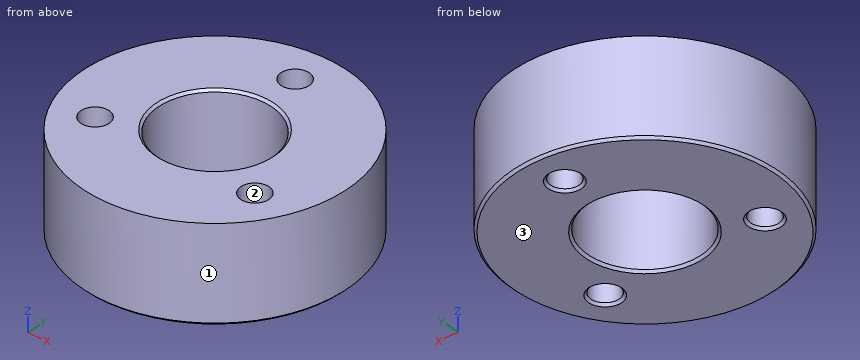
```python
from build123d import *

# Parameters (mm, degrees)
SKETCH2_R           = 14
SKETCH2_R_2         = 6
SKETCH2_R_3         = 1.5
BOSS_EXTRUDE1_DEPTH = 10
CHAMFER1_SIZE       = 0.25


with BuildPart() as part:
    # Sketch2 → Boss-Extrude1 (new body)
    with BuildSketch(Plane.XY):
        Circle(SKETCH2_R)
        Circle(SKETCH2_R_2, mode=Mode.SUBTRACT)
        with Locations((0, 10)):
            Circle(SKETCH2_R_3, mode=Mode.SUBTRACT)
        with Locations((8.660254038, -5)):
            Circle(SKETCH2_R_3, mode=Mode.SUBTRACT)
        with Locations((-8.660254038, -5)):
            Circle(SKETCH2_R_3, mode=Mode.SUBTRACT)
    extrude(amount=BOSS_EXTRUDE1_DEPTH)

    # Chamfer1
    chamfer1_edges = [part.edges().sort_by_distance(p)[0] for p in [
        (7.160254038, -5, 0),
        (-10.160254038, -5, 0),
        (-14, 0, 0),
        (-6, 0, 0),
        (-6, 0, 10),
        (-1.5, 10, 0),
    ]]
    chamfer(chamfer1_edges, length=CHAMFER1_SIZE)


solid = part.part
```
Check sheet for the modelled part. Datum: model origin and axes. Units: mm. Face numbers are marked on the shaded views. Give positions to 0.01 mm unless a question says otherwise; leave off trailing zeros. Order: outer loops, then holes, each group sorted by start corner. A loop starts at its lowest first (then second) coordinate and runs counter-clockwise, first axis right, second up. Notation, with made-up numbers: (-32, 76.5) -> (27, 76.5) arc R23 cw to (27, 90.5) -> close; hole circle Ø4 at (-12, -5). An arc over 180 degrees is marked (long way). Use CSV: the item, a comma, the result in double quotes. Start each with the question number.
1) Material ranges on line 1 (Y direction, x = 0, z = 4.5); line 2 (Y direction, x = -10, z = 1.75); line 3 (X direction, y = 1.5, z = 6), recorded low to high. Write a range as from..to.
2) Sectioned sample at A-A, the plane x = 0. Record the boundary of the cut face in (y, z).
3) Sectioned sample at B-B, the plane y = 0. Record the boundary of the cut face in (x, z), plus the area to 3 significant figures.
4) Sectioned sample at C-C, the plane z = 3.25. Record the boundary of the cut face in (x, y).
5) Sectioned sample at D-D, the plane y = -5. Give the number of separate pieces and of enclosed holes in the cut face, plus the area to 3 significant figures.
6) Mould release check, pull along X, two halves, no side actions. Record for the marked faces 1, 2 and 3: released by +X, released by -X, zero draft, split by the parting line, or undercut.
7) Go/stop test with flat-tipped pins: P1, Ø15.5, axis at x = 0, y = 0, coming from the +Z side; P2, Ø2.5, axis at x = 8.66, y = -5, coming from the +Z side; P3, Ø5, axis at y = -7, z = 3.5, coming from the +X side. Record where each tip stops, or that it passes through.
Recorded:
1,line 1,"-14..-6, 6..8.5, 11.5..14"
1,line 2,"-9.8..-5.67, -4.33..9.8"
1,line 3,"-13.92..-5.81, 5.81..13.92"
2,outline,"(-14, 0.25) -> (-13.75, 0) -> (-6.25, 0) -> (-6, 0.25) -> (-6, 9.75) -> (-6.25, 10) -> (-14, 10) -> close; (6, 0.25) -> (6.25, 0) -> (8.25, 0) -> (8.5, 0.25) -> (8.5, 10) -> (6.25, 10) -> (6, 9.75) -> close; (11.5, 0.25) -> (11.75, 0) -> (13.75, 0) -> (14, 0.25) -> (14, 10) -> (11.5, 10) -> close"
3,outline,"(-14, 0.25) -> (-13.75, 0) -> (-6.25, 0) -> (-6, 0.25) -> (-6, 9.75) -> (-6.25, 10) -> (-14, 10) -> close; (6, 0.25) -> (6.25, 0) -> (13.75, 0) -> (14, 0.25) -> (14, 10) -> (6.25, 10) -> (6, 9.75) -> close"
3,area,"160 mm2"
4,outline,"circle Ø28 at (0, 0); hole circle Ø3 at (-8.66, -5); hole circle Ø12 at (0, 0); hole circle Ø3 at (0, 10); hole circle Ø3 at (8.66, -5)"
5,separate pieces,"4"
5,enclosed holes,"0"
5,area,"135 mm2"
6,face 1,"split by the parting line"
6,face 2,"undercut"
6,face 3,"zero draft"
7,P1,"z = 10"
7,P2,"through"
7,P3,"x = 13.26"
